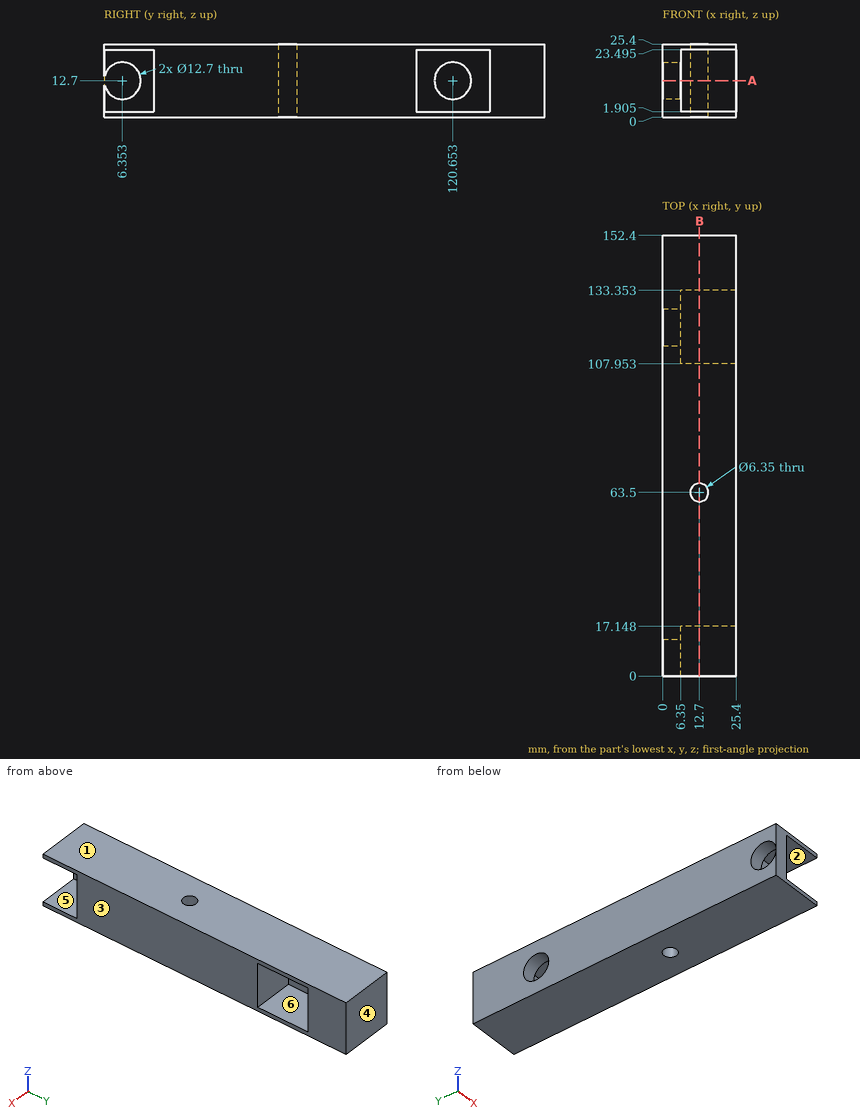
The drawing under review shows one solid part. Ordinate dimensions are in mm from its lowest x, y, z. A direction names the side the tool comes from. Give positions to 0.01 mm unless a question says otherwise; leave off trailing zeros. Write each loop counter-clockwise with the first axis right and the second up, starting at its lowest first coordinate (ties: lowest second). Pieces come first, ordered by that corner, then holes. Notation, with made-up numbers: (-28, 29) - (17, 29) arc R31 ccw to (17, 60) - close; hole circle Ø6 at (15.5, -5). An arc over 180 degrees is marked (long way). Answer in a Markdown table with one row per item. Add a question column.
1. We need section B-B on x = 12.7. Write out the cut boundary in (y, z) (1 decimal).
2. Insertion check: P1, Ø11, axis at y = 125, z = 9, coming from the +X side; P2, Ø1, axis at x = 14.5, z = 12, coming from the -Y side. Each pin has a flat end and moves straight along its axis. Give the tip position at first contact, or say it passes through.
3. Wall thickness on line 1 along Y through (x, z) = (12.7, 13.5) (1 decimal); line 2 along Y through (x, z) = (16.5, 11.25); line 3 along Z through (x, y) = (13, 109) (1 decimal): over which ranges is each line inside the solid? List them lowest first. Write a range as [from, to].
4. Draft analysis for pull direction Z (two halves, no side actions). For the marked faces 1, 2 and 3, state which applies: +Z half, -Z half, draft (parallel to the pull), parting line (faces both ways), or undercut.
5. We need section A-A on z = 12.7. State how many separate pieces and enclosed holes the cut face has, then the cut area to 3 significant figures.
6. Tool access review of the marked faces 4, 5 and 6: name each direction out of +Z, -Z, +X, -X, +Y, -Y from which nothing blocks a thin tool from reaching the whole face with its end or side.
Ans:
| question | item | result |
|---|---|---|
| 1 | outline | (0, 0) - (60.3, 0) - (60.3, 25.4) - (0, 25.4) - (0, 23.5) - (17.1, 23.5) - (17.1, 1.9) - (0, 1.9) - close; (66.7, 0) - (152.4, 0) - (152.4, 25.4) - (66.7, 25.4) - close; hole (108, 1.9) - (133.4, 1.9) - (133.4, 23.5) - (108, 23.5) - close |
| 2 | P1 | stops at x = 6.35 |
| 2 | P2 | stops at y = 17.15 |
| 3 | line 1 | y = [17.1, 60.3], [66.7, 108], [133.4, 152.4] |
| 3 | line 2 | y = [17.15, 107.95], [133.35, 152.4] |
| 3 | line 3 | z = [0, 1.9], [23.5, 25.4] |
| 4 | face 1 | +Z half |
| 4 | face 2 | undercut |
| 4 | face 3 | draft |
| 5 | separate pieces | 3 |
| 5 | enclosed holes | 1 |
| 5 | area | 2,870 mm^2 |
| 6 | face 4 | +Z, -Z, +X, -X, +Y |
| 6 | face 5 | +X, -Y |
| 6 | face 6 | +X |
